Verification items for this drawing (mm, ordinates from the low corner). A direction names the side the tool comes from. Give positions to 0.01 mm unless a question says otherwise; leave off trailing zeros. Write each loop counter-clockwise with the first axis right and the second up, starting at its lowest first coordinate (ties: lowest second). Pieces come first, ordered by that corner, then holes. Notation, with made-up numbers: (-34, 12.5) -> (-2, 12.5) arc R7 cw to (-2, 18.5) -> close; hole circle Ø3 at (52, -11.75). An arc over 180 degrees is marked (long way). Use one line per item in the form item = value. Start each with the question number.
(1) Release check for a two-part mould opening along X. For the marked faces 1, 2, 3 and 4 record: pulls with the +X half, pulls with the -X half, needs draft (parallel to the pull), parting line crosses it, or undercut.
(2) Section check A-A, the plane z = 4. Record the cut outline in (x, y) (1 decimal), plus the area to 3 significant figures.
(3) Scan lines: L1, parallel to Z at x = 36, y = 40; L2, parallel to X at y = 19, z = 4 (1 decimal); L3, parallel to X at y = 86, z = 20 (1 decimal). Record each from-to range of solid material in increasing order.
(4) Section check C-C, the plane y = 50.5. Record the cut outline in (x, z) (1 decimal), plus the area to 3 significant figures.
(5) Depth check by flat-ended pin: pin 1 Ø1 at (x, y) = (30.5, 23) entering from +Z; pin 2 Ø6 at (y, z) = (58, 15) entering from +X; pin 3 Ø8 at (y, z) = (70, 33.5) entering from +X; pin 4 Ø2 at (y, z) = (42, 33) entering from -X. Enter the tip coordinate at first touch or a pass-through.
(6) Section check B-B, the plane x = 30. Record the cut outline in (y, z).
(7) Set-up check for the marked faces 5 and 6: record each of +Z, -Z, +X, -X, +Y, -Y from which the full face is reachable in a straight line by a thin tool's end or side.
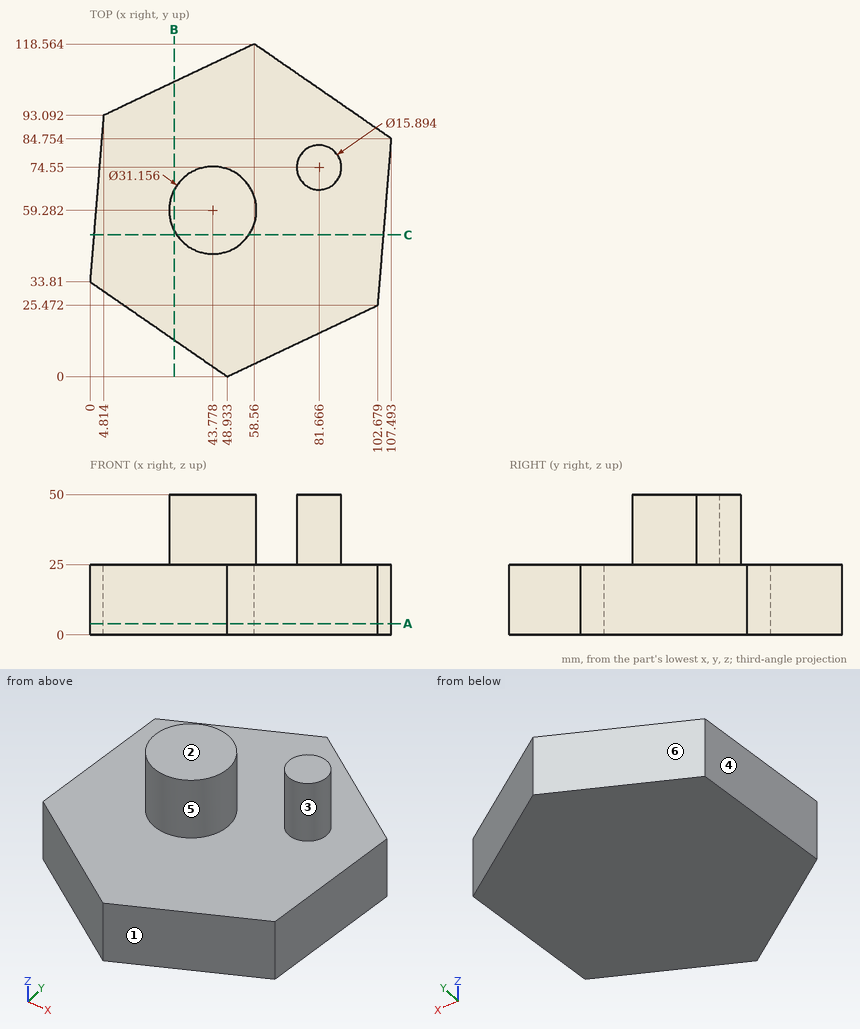
Completed:
q1.face_1 = pulls with the +X half
q1.face_2 = needs draft
q1.face_3 = undercut
q1.face_4 = pulls with the -X half
q2.outline = (0, 33.8) -> (48.9, 0) -> (102.7, 25.5) -> (107.5, 84.8) -> (58.6, 118.6) -> (4.8, 93.1) -> close
q2.area = 9,190 mm²
q3.L1 = 0 to 25
q3.L2 = 21.4 to 89
q3.L3 = 4.2 to 105.7
q4.outline = (1.4, 0) -> (104.7, 0) -> (104.7, 25) -> (56.6, 25) -> (56.6, 50) -> (30.9, 50) -> (30.9, 25) -> (1.4, 25) -> close
q4.area = 3,230 mm²
q5.pin_1 = 25
q5.pin_2 = 105.56
q5.pin_3 = 89.59
q5.pin_4 = through
q6.outline = (13.08, 0) -> (105.03, 0) -> (105.03, 25) -> (66.55, 25) -> (66.55, 50) -> (52.01, 50) -> (52.01, 25) -> (13.08, 25) -> close
q7.face_5 = +Z
q7.face_6 = +Z, -Z, -X, +Y
